Read the model definition and answer for the solid it produces. Units are mm, in the model's axes. A direction names the side the tool comes from. Round coordinates to 2 decimals unless told otherwise and drop trailing zeros. Write each loop counter-clockwise with the first axis right and the second up, starting at its lowest first coordinate (ties: lowest second). Pieces come first, ordered by that corner, then holes. Notation, with made-up numbers: (81.5, 23) -> (111.5, 23) arc R12 ccw to (111.5, 43) -> close; hole circle Ø4 at (61.5, 12). An arc over 180 degrees is marked (long way). Return JSON: item names as keys, results as strings.
from build123d import *

# Parameters (mm, degrees)
F0_W           = 10.16
F0_H           = 19.05
F1_DEPTH       = 3.175
F4_DEPTH       = 10.16
F6_D           = 4.4
F6_DEPTH       = 12.7
F6_CBORE_D     = 8.25
F6_CBORE_DEPTH = 1.27
F7_R           = 25.4
F8_DEPTH       = 1.778


with BuildPart() as f1:
    # F0 (on Top) → F1 (new body)
    with BuildSketch(Plane.XY):
        Rectangle(F0_W, F0_H)
    extrude(amount=F1_DEPTH)

    # F2 (on face) → F4 (join, through all)
    with BuildSketch(Plane.YZ.offset(5.08)):
        Polygon((3.81, 6.35), (1.27, 3.175), (9.525, 3.175), (9.525, 6.35), align=None)
    extrude(amount=-F4_DEPTH)

    # F6
    with Locations(Plane.XY.offset(3.175)):
        with Locations((0, -4.445)):
            CounterBoreHole(F6_D / 2, F6_CBORE_D / 2, F6_CBORE_DEPTH, depth=F6_DEPTH)

    # F7 (on face) → F8 (cut)
    with BuildSketch(Plane.XY.offset(3.175)):
        with Locations((0, 31.75)):
            Circle(F7_R)
    extrude(amount=F8_DEPTH, mode=Mode.SUBTRACT)


solid = f1.part
Item 1: Section A-A (x = 0) is taken. Give the vertices of the cut face in (y, z) (3 decimals).
Worked answers:
{"outline": "(-9.525, 0) -> (-6.645, 0) -> (-6.645, 1.905) -> (-8.57, 1.905) -> (-8.57, 3.175) -> (-9.525, 3.175) -> close; (-2.245, 0) -> (9.525, 0) -> (9.525, 3.175) -> (6.35, 3.175) -> (6.35, 4.953) -> (9.525, 4.953) -> (9.525, 6.35) -> (3.81, 6.35) -> (1.27, 3.175) -> (-0.32, 3.175) -> (-0.32, 1.905) -> (-2.245, 1.905) -> close"}
Item 2: A tool of negligible diameter and unlimited length cuts with its end or side. For faces 5 (the cylindrical face through (-0.07, 6.35, 4.05)), 6 (the flat face through (2, -6, 1.905)), 7 (the flat face through (0, 9.525, 2)), from which of +Z, -Z, +X, -X, +Y, -Y can it reach the whole face along a straight path? Write none if from no direction.
Worked answers:
{"face 5": "+Y", "face 6": "+Z", "face 7": "+Z, -Z, +X, -X, +Y"}
Item 3: Flat-ended cylindrical pins translate along their axes: pin 1 (2.5 mm diameter, centred on x = 1, y = -4.5, fed in from +Z) (3 decimals); pin 2 (2.5 mm diameter, centred on x = 0, y = -4.445, fed in from +Z). Find the tip coordinate at first contact, or state that the pin passes through.
Worked answers:
{"pin 1": "stops at z = 1.905", "pin 2": "passes through"}
Item 4: Section B-B (z = 1.5) is taken. Give the vertices of the cut face in (x, y) (3 decimals), then the cut area to 3 significant figures.
Worked answers:
{"outline": "(-5.08, -9.525) -> (5.08, -9.525) -> (5.08, 9.525) -> (-5.08, 9.525) -> close; hole circle Ø4.4 at (0, -4.445)", "area": "178 mm2"}
Item 5: For a pull along X with two mould halves and no side action, classify faces 1 (the flat face through (-5.08, 2, 3)), 2 (the flat face through (5.08, 2, 3)), 3 (the flat face through (1, 0, 3.175)), 4 (the cylindrical face through (2.198, -4.348, 0.939)) as released by +X, released by -X, zero draft, split by the parting line, or undercut.
Worked answers:
{"face 1": "released by -X", "face 2": "released by +X", "face 3": "zero draft", "face 4": "undercut"}
Item 6: Section C-C (x = -2) is taken. Give the vertices of the cut face in (y, z) (3 decimals), then the cut area to 3 significant figures.
Worked answers:
{"outline": "(-9.525, 0) -> (-5.362, 0) -> (-5.362, 1.905) -> (-8.053, 1.905) -> (-8.053, 3.175) -> (-9.525, 3.175) -> close; (-3.528, 0) -> (9.525, 0) -> (9.525, 3.175) -> (6.429, 3.175) -> (6.429, 4.953) -> (9.525, 4.953) -> (9.525, 6.35) -> (3.81, 6.35) -> (1.27, 3.175) -> (-0.837, 3.175) -> (-0.837, 1.905) -> (-3.528, 1.905) -> close", "area": "64.5 mm2"}
Item 7: Section D-D (z = 4.5) is taken. Give the vertices of the cut face in (x, y), then the cut area to 3 significant figures.
Worked answers:
{"outline": "(-5.08, 2.33) -> (5.08, 2.33) -> (5.08, 6.86) arc R25.4 cw to (-5.08, 6.86) -> close", "area": "42.6 mm2"}
Item 8: Straight lines are drawn through the part: L1, parallel to Y at x = 0, z = 2.45 (3 decimals); L2, parallel to Y at x = 0, z = 1.45 (3 decimals); L3, parallel to Z at x = -1, y = -1.75 (3 decimals). For each, find the intervals that lie inside material, in ascending order. Write a range as [from, to].
Worked answers:
{"L1": "y = [-9.525, -8.57], [-0.32, 9.525]", "L2": "y = [-9.525, -6.645], [-2.245, 9.525]", "L3": "z = [0, 1.905]"}
